Geometry: see drawing. Coordinates: mm, zero at the bounding-box minimum. A direction names the side the tool comes from. Give positions to 0.01 mm unless a question says otherwise; leave off trailing zeros. Loops run counter-clockwise (first coordinate to the right, second up) from the corner with the lowest first, then second, coordinate; pieces in that order, holes last. Notation, with made-up numbers: (46.5, 60) -> (86.5, 60) arc R20 ccw to (86.5, 64) -> close; hole circle Ø3 at (30, 49.5). An arc over 180 degrees is marked (long way). Return JSON: item names as keys, results as strings. Group by question number.
(1) Ray query, line 1 (Y direction, x = 84.5, z = 20) (1 decimal); line 2 (Y direction, x = 21, z = 53) (1 decimal); line 3 (X direction, y = 57, z = 13.5). Return the intervals inside material, ascending. Write a range as from..to.
(2) Cut plane D-D on z = 65. Return loops of the section in (x, y) (1 decimal).
(3) Pin query (flat end, axial travel): pin 1 (2 mm diameter, centred on x = 99.5, y = 17, fed in from -Z); pin 2 (23.5 mm diameter, centred on x = 118, y = 47, fed in from +Z). Return the tip coordinate at first contact, or that it passes through.
(4) Draft query along Y for the marked faces 1, 2 and 3. Return one class per face: released by +Y, released by -Y, zero draft, split by the parting line, or undercut.
(5) Cut plane A-A on z = 8. Return loops of the section in (x, y) (1 decimal), then the cut area to 3 significant figures.
(6) Access query for the marked faces 4, 5 and 6. Directions: +Z, -Z, +X, -X, +Y, -Y. A direction counts if a zero-diameter tool reaches every point of the face in a straight line with its end or side. Return the directions, or none.
(7) Cut plane B-B on y = 80.5. Return loops of the section in (x, z).
(8) Cut plane C-C on x = 88. Return loops of the section in (y, z) (1 decimal), then the cut area to 3 significant figures.
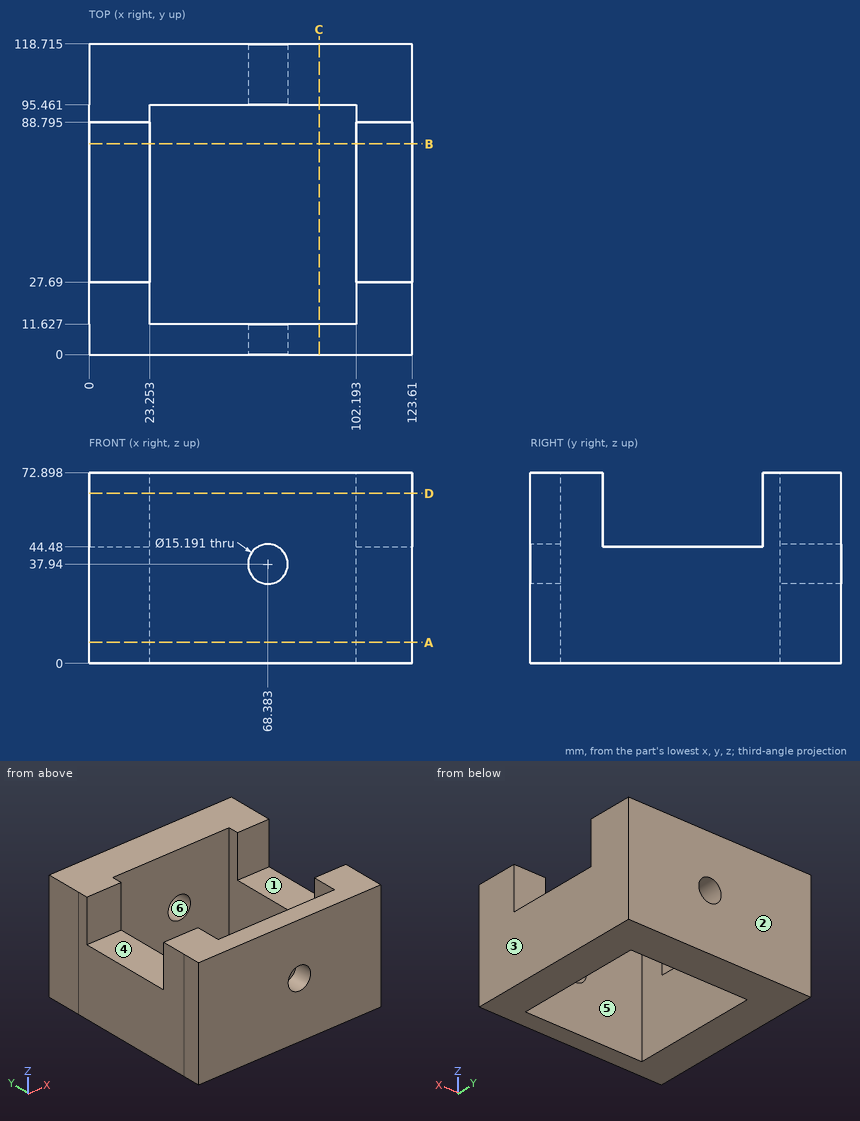
Answers:
{
 "1": {"line 1": "0..11.6, 95.5..118.7", "line 2": "0..27.7, 88.8..118.7", "line 3": "0..23.25, 102.19..123.61"},
 "2": {"outline": "(0, 0) -> (123.6, 0) -> (123.6, 27.7) -> (102.2, 27.7) -> (102.2, 11.6) -> (23.3, 11.6) -> (23.3, 27.7) -> (0, 27.7) -> close; (0, 88.8) -> (23.3, 88.8) -> (23.3, 95.5) -> (102.2, 95.5) -> (102.2, 88.8) -> (123.6, 88.8) -> (123.6, 118.7) -> (0, 118.7) -> close"},
 "3": {"pin 1": "through", "pin 2": "z = 44.48"},
 "4": {"face 1": "undercut", "face 2": "released by +Y", "face 3": "zero draft"},
 "5": {"outline": "(0, 0) -> (123.6, 0) -> (123.6, 118.7) -> (0, 118.7) -> close; hole (23.3, 11.6) -> (102.2, 11.6) -> (102.2, 95.5) -> (23.3, 95.5) -> close", "area": "8,060 mm²"},
 "6": {"face 4": "+Z, +X, -X", "face 5": "+Z, -Z", "face 6": "+Y, -Y"},
 "7": {"outline": "(0, 0) -> (23.25, 0) -> (23.25, 44.48) -> (0, 44.48) -> close; (102.19, 0) -> (123.61, 0) -> (123.61, 44.48) -> (102.19, 44.48) -> close"},
 "8": {"outline": "(0, 0) -> (11.6, 0) -> (11.6, 72.9) -> (0, 72.9) -> close; (95.5, 0) -> (118.7, 0) -> (118.7, 72.9) -> (95.5, 72.9) -> close", "area": "2,540 mm²"}
}
